Design review of the part built by this model. Coordinates are the model's own, in mm. Face numbers are marked on the shaded views. A direction names the side the tool comes from. Coordinates: 2 decimals unless noted, no trailing zeros. Loops run counter-clockwise (first coordinate to the right, second up) from the corner with the lowest first, then second, coordinate; pieces in that order, holes last.
Q1. Draft analysis for pull direction Y (two halves, no side actions). For the marked faces 4, 5 and 6, state which applies: released by +Y, released by -Y, zero draft, split by the parting line, or undercut.
Q2. For P1, Ø12, axis at x = 84, z = 6, coming from the +Y side; P2, Ø4, axis at x = -28.5, z = 9.5, coming from the -Y side; P3, Ø2, axis at y = -10, z = 8.5, coming from the +X side, all flat-tipped, find the tip position at first contact; note any pin that passes through.
Q3. Machinability: for the marked faces 1, 2 and 3, which of the approach directions +Z, -Z, +X, -X, +Y, -Y give a long, thin tool a straight path to every point of the face, cutting with its end or side? Answer none if there is none.
Q4. Add section B-B on x = 20. Give the boundary of the cut face in (y, z).
Q5. Add section D-D on x = 53. Give the boundary of the cut face in (y, z).
Q6. Wall thickness on probe 1 along X at (y, z) = (-21.5, 15.25); probe 2 along Y at (x, z) = (4, 7); probe 3 along Y at (x, z) = (-20, 5.25): over which ranges is each line inside the solid? List them lowest first.
Q7. Add section A-A on x = -86. Give the boundary of the cut face in (y, z).
Q8. Add section C-C on y = -67. Give the boundary of the cut face in (x, z).
```python
from build123d import *

# Parameters (mm, degrees)
BOSS_EXTRUDE1_DEPTH = 20
FILLET1_R           = 10


with BuildPart() as part:
    # Sketch2 → Boss-Extrude1 (new body)
    with BuildSketch(Plane.XY):
        with BuildLine():
            Line((8.524308176, 123.574202785), (34.312591702, 119.949895893))
            Line((34.312591702, 119.949895893), (30.946870999, 113.619895893))
            ThreePointArc((30.946870999, 113.619895893), (29.437456237, 96.527152904), (40.66334756, 83.549496728))
            Line((40.66334756, 83.549496728), (74.333931823, 66.991594994))
            Line((74.333931823, 66.991594994), (111.389403677, 43.150824518))
            ThreePointArc((111.389403677, 43.150824518), (117.222239734, 37.405423132), (120.264178278, 29.804224315))
            Line((120.264178278, 29.804224315), (124.786275456, 4.158136801))
            Line((124.786275456, 4.158136801), (117.726022813, 5.403049832))
            ThreePointArc((117.726022813, 5.403049832), (101.003423398, 1.556640514), (92.129930121, -13.130132886))
            Line((92.129930121, -13.130132886), (86.787212529, -50.269434484))
            Line((86.787212529, -50.269434484), (75.564062952, -92.878485691))
            ThreePointArc((75.564062952, -92.878485691), (71.902306992, -100.201269099), (65.613148031, -105.443224185))
            Line((65.613148031, -105.443224185), (42.619674262, -117.669071055))
            Line((42.619674262, -117.669071055), (41.621918861, -110.569672489))
            ThreePointArc((41.621918861, -110.569672489), (32.796198806, -95.854141193), (16.086187039, -91.953410163))
            Line((16.086187039, -91.953410163), (-20.886378289, -98.348859135))
            Line((-20.886378289, -98.348859135), (-64.878138042, -100.841930533))
            ThreePointArc((-64.878138042, -100.841930533), (-72.974063741, -99.622258186), (-79.902916283, -95.26076578))
            Line((-79.902916283, -95.26076578), (-98.635761771, -77.170667172))
            Line((-98.635761771, -77.170667172), (-92.192155877, -74.02791059))
            ThreePointArc((-92.192155877, -74.02791059), (-80.924151432, -61.086802768), (-82.37801338, -43.989245011))
            Line((-82.37801338, -43.989245011), (-99.885597812, -10.802548251))
            Line((-99.885597812, -10.802548251), (-115.850850987, 30.265700095))
            ThreePointArc((-115.850850987, 30.265700095), (-117.19265228, 38.342282469), (-115.185759692, 46.279788104))
            Line((-115.185759692, 46.279788104), (-103.76982114, 69.685930773))
            Line((-103.76982114, 69.685930773), (-98.789698287, 64.528862593))
            ThreePointArc((-98.789698287, 64.528862593), (-82.999968499, 57.811375783), (-67.188492831, 64.477516571))
            Line((-67.188492831, 64.477516571), (-41.036209743, 91.383472116))
            Line((-41.036209743, 91.383472116), (-6.911519091, 119.25811685))
            ThreePointArc((-6.911519091, 119.25811685), (0.355127803, 123.030046924), (8.524308176, 123.574202785))
        make_face()
        Polygon((-11.954339629, -44.614202866), (32.659863237, -32.659863237), (44.614202866, 11.954339629), (11.954339629, 44.614202866), (-32.659863237, 32.659863237), (-44.614202866, -11.954339629), align=None, mode=Mode.SUBTRACT)
    extrude(amount=BOSS_EXTRUDE1_DEPTH)

    # Fillet1
    fillet1_edges = [part.edges().sort_by_distance(p)[0] for p in [
        (-44.614202866, -11.954339629, 10),
        (-11.954339629, -44.614202866, 10),
        (32.659863237, -32.659863237, 10),
        (44.614202866, 11.954339629, 10),
        (11.954339629, 44.614202866, 10),
        (-32.659863237, 32.659863237, 10),
    ]]
    fillet(fillet1_edges, radius=FILLET1_R)


solid = part.part
```
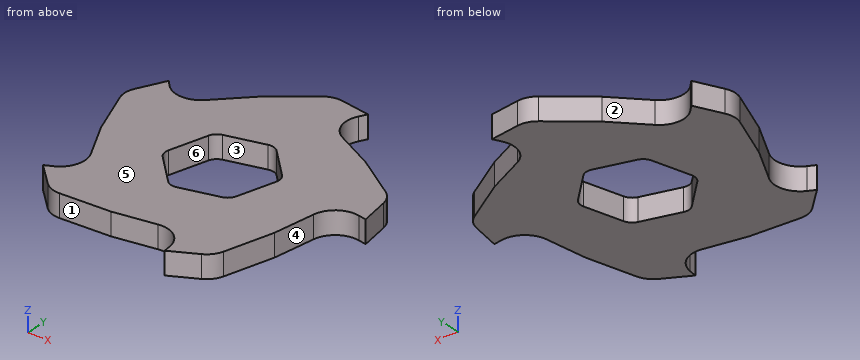
Entries:
1. face 4: released by -Y
1. face 5: zero draft
1. face 6: undercut
2. P1: stops at y = 64.63
2. P2: stops at y = -98.89
2. P3: stops at x = 93.14
3. face 1: +Z, -Z, -Y
3. face 2: +Z, -Z, +Y
3. face 3: +Z, -Z
4. outline: (-91.63, 0) - (-36.05, 0) - (-36.05, 20) - (-91.63, 20) - close; (36.57, 0) - (121.96, 0) - (121.96, 20) - (36.57, 20) - close
5. outline: (-112.15, 0) - (77.48, 0) - (77.48, 20) - (-112.15, 20) - close
6. probe 1: x = -94.24 to -35.07, 35.65 to 90.93
6. probe 2: y = -94.04 to -40.34, 42.48 to 123.69
6. probe 3: y = -98.2 to -36.57, 36.05 to 108.57
7. outline: (-89.37, 0) - (-69.53, 0) - (-69.53, 20) - (-89.37, 20) - close; (-37.12, 0) - (58.02, 0) - (58.02, 20) - (-37.12, 20) - close
8. outline: (-83.9, 0) - (82.38, 0) - (82.38, 20) - (-83.9, 20) - close
